```python
from build123d import *

# Parameters (mm, degrees)
F0_W     = 26.67
F0_H     = 40
F0_W_2   = 13.33
F0_W_3   = 40
F1_DEPTH = 40


with BuildPart() as f1:
    # F0 (on Front) → F1 (new body)
    with BuildSketch(Plane.XZ):
        with Locations((-33.335, 80)):
            Rectangle(F0_W, F0_H)
        with Locations((-13.335, 80)):
            Rectangle(F0_W_2, F0_H)
        with Locations((13.335, 80)):
            Rectangle(F0_W_2, F0_H)
        with Locations((33.335, 80)):
            Rectangle(F0_W, F0_H)
        Polygon((-60, 20), (-20, 20), (-20, 60), (-46.67, 60), (-60, 60), align=None)
        Polygon((20, 20), (20, 60), (6.67, 60), (-6.67, 60), (-20, 60), (-20, 20), align=None)
        Polygon((60, 20), (60, 60), (46.67, 60), (20, 60), (20, 20), align=None)
        with Locations((40, 0)):
            Rectangle(F0_W_3, F0_H)
        with Locations((40, -40)):
            Rectangle(F0_W_3, F0_H)
        with Locations((40, -80)):
            Rectangle(F0_W_3, F0_H)
        with Locations((0, -80)):
            Rectangle(F0_W_3, F0_H)
        with Locations((-40, -80)):
            Rectangle(F0_W_3, F0_H)
        with Locations((-40, -40)):
            Rectangle(F0_W_3, F0_H)
        with Locations((-40, 0)):
            Rectangle(F0_W_3, F0_H)
    extrude(amount=F1_DEPTH)


solid = f1.part
```
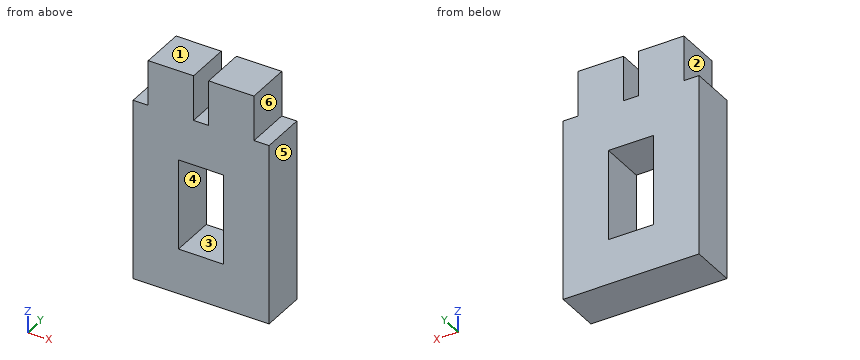
The listing builds one solid part. Answer for the finished solid, in the listing's coordinates (mm). Face numbers are marked on the shaded views. A direction names the side the tool comes from. Give positions to 0.01 mm unless a question says otherwise; leave off trailing zeros. Order: outer loops, then holes, each group sorted by start corner. A loop starts at its lowest first (then second) coordinate and runs counter-clockwise, first axis right, second up. Notation, with made-up numbers: (24.25, 35.5) - (34.25, 35.5) arc R26 cw to (34.25, 61.5) - close; hole circle Ø10 at (-11, 54). An arc over 180 degrees is marked (long way). Use one line per item in the form item = value. Start each with the question number.
(1) A cutting plane is placed at D-D, the plane x = 52.5. Write down the section's boundary in (y, z).
(2) The mould has two halves that part along X. Classify the marked faces 1, 2 and 3: released by +X, released by -X, zero draft, split by the parting line, or undercut.
(3) A cutting plane is placed at C-C, the plane z = -48. Write down the section's boundary in (x, y), then the cut area to 3 significant figures.
(4) For the marked faces 4, 5 and 6, determine the directions among +Z, -Z, +X, -X, +Y, -Y from which every point of the face is accessible in a straight line to the end or side of a thin tool.
(5) A cutting plane is placed at B-B, the plane y = -20. Write down the section's boundary in (x, z).
(6) Flat-ended cylindrical pins translate along their axes: pin 1 Ø6.5 at (x, y) = (1, -10.5) entering from +Z; pin 2 Ø20 at (y, z) = (-17, 71.5) entering from +X; pin 3 Ø20 at (y, z) = (-12, 75.5) entering from -X. Find the tip coordinate at first contact, or state that the pin passes through.
(7) Consider line 1 (Z direction, x = -6.5, y = -3); line 2 (X direction, y = -12, z = 80.5); line 3 (X direction, y = -6, z = -53). Determine where each line is inside the solid, lowest interval first. Write a range as from..to.
(8) A cutting plane is placed at A-A, the plane x = -17. Write down the section's boundary in (y, z).
Ans:
q1.outline = (-40, -100) - (0, -100) - (0, 60) - (-40, 60) - close
q2.face_1 = zero draft
q2.face_2 = released by -X
q2.face_3 = undercut
q3.outline = (-60, -40) - (-20, -40) - (-20, 0) - (-60, 0) - close; (20, -40) - (60, -40) - (60, 0) - (20, 0) - close
q3.area = 3,200 mm^2
q4.face_4 = +Y, -Y
q4.face_5 = +Z, -Z, +X, +Y, -Y
q4.face_6 = +Z, +X, +Y, -Y
q5.outline = (-60, -100) - (60, -100) - (60, 60) - (46.67, 60) - (46.67, 100) - (6.67, 100) - (6.67, 60) - (-6.67, 60) - (-6.67, 100) - (-46.67, 100) - (-46.67, 60) - (-60, 60) - close; hole (-20, -60) - (20, -60) - (20, 20) - (-20, 20) - close
q6.pin_1 = 60
q6.pin_2 = 46.67
q6.pin_3 = -46.67
q7.line_1 = -100..-60, 20..60
q7.line_2 = -46.67..-6.67, 6.67..46.67
q7.line_3 = -60..-20, 20..60
q8.outline = (-40, -100) - (0, -100) - (0, -60) - (-40, -60) - close; (-40, 20) - (0, 20) - (0, 100) - (-40, 100) - close
